Input: part model. Units: mm. Frame: model coordinates. A direction names the side the tool comes from. Give positions to 0.01 mm unless a question says otherwise; leave off trailing zeros. Loops run counter-clockwise (first coordinate to the right, second up) from the corner with the lowest first, then second, coordinate; pieces in that order, holes last. Notation, with made-up numbers: M -7,67.25 L 1,67.25 A24 ccw 1,101.25 Z; hole C 27.5,55.25 d9. An arc over 180 degrees is marked long. Return JSON: item names as keys, results as strings. Group by question number.
```python
from build123d import *

# Parameters (mm, degrees)
SKETCH1_W           = 25.4
SKETCH1_H           = 76.2
BOSS_EXTRUDE1_DEPTH = 88.9
SHELL1_T            = -3.175
SKETCH2_W           = 25.4
SKETCH2_H           = 25.4
CUT_EXTRUDE1_DEPTH  = 26.4
SKETCH3_R           = 2.38125
CUT_EXTRUDE2_DEPTH  = 77.2
SKETCH5_R           = 12.7
CUT_EXTRUDE3_DEPTH  = 26.4


with BuildPart() as part:
    # Sketch1 → Boss-Extrude1 (new body, symmetric)
    with BuildSketch(Plane.XY):
        Rectangle(SKETCH1_W, SKETCH1_H)
    extrude(amount=BOSS_EXTRUDE1_DEPTH, both=True)

    # Shell1
    shell1_openings = [part.faces().sort_by_distance(p)[0] for p in [
        (0, 0, 88.9),
        (0, 0, -88.9),
    ]]
    offset(amount=SHELL1_T, openings=shell1_openings, kind=Kind.INTERSECTION)

    # Sketch2 → Cut-Extrude1 (cut, through all)
    with BuildSketch(Plane.ZY.offset(12.7)):
        with Locations((-76.2, 25.4)):
            Rectangle(SKETCH2_W, SKETCH2_H)
    extrude(amount=-CUT_EXTRUDE1_DEPTH, mode=Mode.SUBTRACT)

    # Sketch3 → Cut-Extrude2 (cut, through all)
    with BuildSketch(Plane(origin=(0, 38.1, 0), x_dir=(1, 0, 0), z_dir=(0, 1, 0))):
        with Locations((0, -88.9)):
            Circle(SKETCH3_R)
        with Locations((0, -75.995900078)):
            Circle(SKETCH3_R)
        with Locations((0, -63.397337518)):
            Circle(SKETCH3_R)
        with Locations((0, -50.731481722)):
            Circle(SKETCH3_R)
        with Locations((0, -38.048590908)):
            Circle(SKETCH3_R)
        with Locations((0, 63.5)):
            Circle(SKETCH3_R)
        with Locations((0, 12.648590908)):
            Circle(SKETCH3_R)
        with Locations((0, 25.331481722)):
            Circle(SKETCH3_R)
        with Locations((0, 37.997337518)):
            Circle(SKETCH3_R)
        with Locations((0, 50.595900078)):
            Circle(SKETCH3_R)
    extrude(amount=-CUT_EXTRUDE2_DEPTH, mode=Mode.SUBTRACT)

    # Sketch5 → Cut-Extrude3 (cut, through all)
    with BuildSketch(Plane(origin=(12.7, 0, 0), x_dir=(0, 0, -1), z_dir=(1, 0, 0))):
        with Locations((20.760556689, 0)):
            Circle(SKETCH5_R)
        with Locations((-38.84233187, 0)):
            Circle(SKETCH5_R)
    extrude(amount=-CUT_EXTRUDE3_DEPTH, mode=Mode.SUBTRACT)


solid = part.part
```
Item 1: Section A-A, the plane x = -5. Return loops of the section in (y, z) (3 decimals).
Item 2: Section D-D, the plane y = 21. Return loops of the section in (x, z) (3 decimals).
Item 3: First-contact query: pin 1 Ø4 at (x, z) = (0, -50.6) entering from +Y; pin 2 Ø5 at (x, y) = (-7.5, 26) entering from -Z. Flat tips, straight axial feed; report the tip coordinate or a pass-through.
Item 4: Pull-direction query (Y, two-part tool) for faces 3 (the face through (11, 12.7, -76)), 4 (the face through (11, 0, 88.9)), 5 (the face through (0, -34.925, 1)), 6 (the face through (-9.525, 0, 1)); classes: pulls with the +Y half, pulls with the -Y half, needs draft (parallel to the pull), parting line crosses it, or undercut.
Item 5: Section B-B, the plane z = 11. Return loops of the section in (x, y) (3 decimals).
Item 6: Section C-C, the plane y = 0. Return loops of the section in (x, z) (3 decimals), then the cut area to 3 significant figures.
Item 7: Reachability of faces 1 (the face through (0, 34.925, 14)), 2 (the face through (-11.09, -7.73, 48.92)) from +Z, -Z, +X, -X, +Y, -Y: full face, straight path, thin tool, end or side. Return the list, or none.
Item 8: Material intervals for line 1 (X direction, y = 29, z = -26) (3 decimals); line 2 (Y direction, x = -4.75, z = -34.5) (3 decimals); line 3 (Z direction, x = 10.5, y = 29.5), sorted ascending. Write a range as from..to.
Answer below:
{
 "1": {"outline": "M -38.1,-88.9 L -34.925,-88.9 L -34.925,88.9 L -38.1,88.9 Z; M 34.925,-63.5 L 38.1,-63.5 L 38.1,88.9 L 34.925,88.9 Z"},
 "2": {"outline": "M -12.7,-63.5 L -9.525,-63.5 L -9.525,88.9 L -12.7,88.9 Z; M 9.525,-63.5 L 12.7,-63.5 L 12.7,88.9 L 9.525,88.9 Z"},
 "3": {"pin 1": "through", "pin 2": "z = -63.5"},
 "4": {"face 3": "pulls with the +Y half", "face 4": "needs draft", "face 5": "undercut", "face 6": "undercut"},
 "5": {"outline": "M -12.7,-38.1 L 12.7,-38.1 L 12.7,38.1 L -12.7,38.1 Z; hole M -9.525,-34.925 L 9.525,-34.925 L 9.525,34.925 L -9.525,34.925 Z"},
 "6": {"outline": "M -12.7,-88.9 L -9.525,-88.9 L -9.525,-33.461 L -12.7,-33.461 Z; M -12.7,-8.061 L -9.525,-8.061 L -9.525,26.142 L -12.7,26.142 Z; M -12.7,51.542 L -9.525,51.542 L -9.525,88.9 L -12.7,88.9 Z; M 9.525,-88.9 L 12.7,-88.9 L 12.7,-33.461 L 9.525,-33.461 Z; M 9.525,-8.061 L 12.7,-8.061 L 12.7,26.142 L 9.525,26.142 Z; M 9.525,51.542 L 12.7,51.542 L 12.7,88.9 L 9.525,88.9 Z", "area": "806 mm^2"},
 "7": {"face 1": "+Z, -Z", "face 2": "+X, -X"},
 "8": {"line 1": "-12.7..-9.525, 9.525..12.7", "line 2": "-38.1..-34.925, 34.925..38.1", "line 3": "-63.5..88.9"}
}
